```python
from build123d import *

# Parameters (mm, degrees)
SKETCH1_R           = 1.5
BOSS_EXTRUDE1_DEPTH = 1
BOSS_EXTRUDE2_START = -2
SKETCH3_R           = 1.5
BOSS_EXTRUDE2_DEPTH = 3.6
CHAMFER1_SIZE       = 0.2
FILLET1_R           = 0.6


with BuildPart() as part:
    # Sketch1 → Boss-Extrude1 (new, symmetric)
    with BuildSketch(Plane(origin=(0, 0, 0), x_dir=(1, 0, 0), z_dir=(0, 1, 0))):
        Polygon((3.175426481, 0), (1.58771324, 2.75), (-1.58771324, 2.75), (-3.175426481, 0), (-1.58771324, -2.75), (1.58771324, -2.75), align=None)
        with Locations(Location((0, 0, 0), (0, 0, 270))):
            Circle(SKETCH1_R, mode=Mode.SUBTRACT)
    extrude(amount=BOSS_EXTRUDE1_DEPTH, both=True)

    # Sketch2 → Cut-Revolve1 (revolve, cut)
    with BuildSketch(Plane.XY):
        with BuildLine():
            Line((-3.55, -0.2), (-3.55, -1))
            Line((-3.55, -1), (-2.75, -1))
            ThreePointArc((-2.75, -1), (-3.315685425, -0.765685425), (-3.55, -0.2))
        make_face()
    cut_revolve1 = revolve(axis=Axis((0, 0, 0), (0, 1, 0)), mode=Mode.SUBTRACT)

    # Mirror2: Cut-Revolve1 across plane
    add(cut_revolve1.mirror(Plane.ZX), mode=Mode.SUBTRACT)

    # Sketch3 → Boss-Extrude2 (add)
    with BuildSketch(Plane(origin=(0, 1, 0), x_dir=(1, 0, 0), z_dir=(0, 1, 0)).offset(BOSS_EXTRUDE2_START)):
        with BuildLine():
            ThreePointArc((-2.38156986, -1.375), (-1.375, -2.38156986), (0, -2.75))
            ThreePointArc((0, -2.75), (1.375, -2.38156986), (2.38156986, -1.375))
            ThreePointArc((2.38156986, -1.375), (2.75, 0), (2.38156986, 1.375))
            ThreePointArc((2.38156986, 1.375), (1.375, 2.38156986), (0, 2.75))
            ThreePointArc((0, 2.75), (-1.375, 2.38156986), (-2.38156986, 1.375))
            ThreePointArc((-2.38156986, 1.375), (-2.75, 0), (-2.38156986, -1.375))
        make_face()
        with Locations(Location((0, 0, 0), (0, 0, 270))):
            Circle(SKETCH3_R, mode=Mode.SUBTRACT)
    extrude(amount=BOSS_EXTRUDE2_DEPTH)

    # Chamfer1
    chamfer1_edges = [part.edges().sort_by_distance(p)[0] for p in [
        (0, -1, -1.5),
    ]]
    chamfer(chamfer1_edges, length=CHAMFER1_SIZE)

    # Fillet1
    fillet1_edges = [part.edges().sort_by_distance(p)[0] for p in [
        (0, 2.6, 2.75),
        (0, 2.6, -1.5),
    ]]
    fillet(fillet1_edges, radius=FILLET1_R)


solid = part.part
```
Geometry: final body of the model. Coordinates: model frame, mm. Coordinates: 2 decimals unless noted, no trailing zeros. Loops run counter-clockwise (first coordinate to the right, second up) from the corner with the lowest first, then second, coordinate; pieces in that order, holes last. Notation, with made-up numbers: M 85,-30 L 119,-30 A13 ccw 119,-9 Z; hole C -2.75,-7 d10. An arc over 180 degrees is marked long. Put each result on its own line as item: value.
(1) Cut plane B-B on y = 1.65. Return the cut outline in (x, z) (3 decimals).
Answer sheet:
outline: C 0,0 d5.5; hole C 0,0 d3
(2) Material intervals for probe 1 along X at (y, z) = (-0.35, 1.15); probe 2 along X at (y, z) = (0.15, 0.95); probe 3 along Z at (x, y) = (-1.25, 0.5), sorted ascending.
Answer sheet:
probe 1: x = -2.51 to -0.96, 0.96 to 2.51
probe 2: x = -2.63 to -1.16, 1.16 to 2.63
probe 3: z = -2.75 to -0.83, 0.83 to 2.75
(3) Draft query along X for faces 1 (the face through (2, -1, 0)), 2 (the face through (0.45, 0.58, 1.43)), 3 (the face through (2.37, 0.014, 1.394)), 4 (the face through (-2.39, 0.01, 1.36)). Return one class per face: pulls with the +X half, pulls with the -X half, needs draft (parallel to the pull), parting line crosses it, or undercut.
Answer sheet:
face 1: needs draft
face 2: undercut
face 3: pulls with the +X half
face 4: pulls with the -X half
(4) Cut plane A-A on y = 0.8. Return the cut outline in (x, z), then the cut area to 3 significant figures.
Answer sheet:
outline: M -3.18,0 L -1.59,-2.75 L 1.59,-2.75 L 3.18,0 L 1.59,2.75 L -1.59,2.75 Z; hole C 0,0 d3
area: 19.1 mm^2
(5) First-contact query: pin 1 (2.5 mm diameter, centred on x = 0, z = 0, fed in from -Y). Flat tip, straight axial feed; report the tip coordinate or a pass-through.
Answer sheet:
pin 1: passes through
